```python
from build123d import *

# Parameters (mm, degrees)
F0_W     = 60
F0_H     = 60
F0_W_2   = 50
F0_H_2   = 50
F1_DEPTH = 1207
F3_DEPTH = 60.001
F5_R     = 49
F6_DEPTH = 118


with BuildPart() as f1:
    # F0 (on Front) → F1 (new body)
    with BuildSketch(Plane.XZ):
        Rectangle(F0_W, F0_H)
        Rectangle(F0_W_2, F0_H_2, mode=Mode.SUBTRACT)
    extrude(amount=F1_DEPTH)

    # F2 (on face) → F3 (cut, through all)
    with BuildSketch(Plane.YZ.offset(30)):
        Polygon((-1207, 30), (-1207, -30), (-1147, 30), align=None)
        Polygon((0, -30), (0, 30), (-60, 30), align=None)
    extrude(amount=-F3_DEPTH, mode=Mode.SUBTRACT)

    # F5 (on face) → F6 (cut, symmetric)
    with BuildSketch(Plane(origin=(0, -45, 45), x_dir=(-1, 0, 0), z_dir=(0, 0.7071067812, -0.7071067812))):
        with Locations((0, 17.5233952504)):
            Circle(F5_R)
    extrude(amount=F6_DEPTH, both=True, mode=Mode.SUBTRACT)


solid = f1.part
```
Geometry: final body of the model. Coordinates: model frame, mm. A direction names the side the tool comes from. Round coordinates to 2 decimals unless told otherwise and drop trailing zeros. Loops run counter-clockwise (first coordinate to the right, second up) from the corner with the lowest first, then second, coordinate; pieces in that order, holes last. Notation, with made-up numbers: (-10, -23) -> (49, -23) arc R13 cw to (49, 0) -> close; hole circle Ø8 at (76.5, 61.5). An arc over 180 degrees is marked (long way). Write each question's results on one line, items separated by ' | '.
Item 1: Cut plane B-B on y = -519. Return the cut outline in (x, z), and give its area (3 significant figures).
Answers below:
outline: (-30, -30) -> (30, -30) -> (30, 30) -> (-30, 30) -> close; hole (-25, -25) -> (25, -25) -> (25, 25) -> (-25, 25) -> close | area: 1,100 mm²
Item 2: Cut plane A-A on x = 14. Return the cut outline in (y, z).
Answers below:
outline: (-1207, -30) -> (-11.63, -30) -> (-16.63, -25) -> (-1202, -25) -> close; (-1152, 25) -> (-66.63, 25) -> (-71.63, 30) -> (-1147, 30) -> close
Item 3: Pull-direction query (Z, two-part tool) for faces 1 (the face through (-30, -595, 0)), 2 (the face through (0, -598, 25)), 3 (the face through (0, -596, 30)); classes: pulls with the +Z half, pulls with the -Z half, needs draft (parallel to the pull), parting line crosses it, or undercut.
Answers below:
face 1: needs draft | face 2: undercut | face 3: pulls with the +Z half
Item 4: Set-up query: faces 4 (the face through (-25, -598, 0)), 5 (the face through (25.191, -33.817, -0.839)). Return all of +Z, -Z, +X, -X, +Y, -Y with unobstructed straight access to the full face (end or side cutting, diameter ignored); none if empty.
Answers below:
face 4: +Y, -Y | face 5: +Z, +Y
Item 5: Line query: probe 1 along X at (y, z) = (-1129.5, -20); probe 2 along X at (y, z) = (-56, 23). Output: solid intervals per line, ascending. Write a range as [from, to].
Answers below:
probe 1: x = [-30, -25], [25, 30] | probe 2: x = [-30, -27.05], [27.05, 30]
